CAD build for the part. Positions are in the model's coordinates, mm. A direction names the side the tool comes from. Coordinates: 2 decimals unless noted, no trailing zeros. Order: outer loops, then holes, each group sorted by start corner. A loop starts at its lowest first (then second) coordinate and runs counter-clockwise, first axis right, second up. Notation, with made-up numbers: M -31.75,88 L 1.25,88 A11 cw 1.25,98 Z; hole C 80,22 d8. An arc over 180 degrees is marked long. Write item = value, one per line. Start each with the question number.
```python
from build123d import *

# Parameters (mm, degrees)
SKETCH1_W           = 170
SKETCH1_H           = 120
BOSS_EXTRUDE1_DEPTH = 10
SKETCH2_W           = 60
SKETCH2_H           = 40
BOSS_EXTRUDE2_DEPTH = 2
SKETCH3_W           = 60
SKETCH3_H           = 8
BOSS_EXTRUDE3_DEPTH = 25
SKETCH4_R           = 1.6
CUT_EXTRUDE1_DEPTH  = 10
CUT_EXTRUDE2_DEPTH  = 36
CHAMFER1_SIZE       = 12
FILLET4_R           = 4
CHAMFER2_SIZE       = 3
CUT_EXTRUDE4_DEPTH  = 5
CUT_EXTRUDE5_DEPTH  = 19
FILLET5_R           = 10
CUT_EXTRUDE6_DEPTH  = 91
FILLET6_R           = 10


with BuildPart() as part:
    # Sketch1 → Boss-Extrude1 (new body)
    with BuildSketch(Plane(origin=(0, 0, 0), x_dir=(1, 0, 0), z_dir=(0, 1, 0))):
        with Locations((85, 60)):
            Rectangle(SKETCH1_W, SKETCH1_H)
    extrude(amount=BOSS_EXTRUDE1_DEPTH)

    # Sketch2 → Boss-Extrude2 (add)
    with BuildSketch(Plane(origin=(0, 10, 0), x_dir=(1, 0, 0), z_dir=(0, 1, 0))):
        with Locations((140, 100)):
            Rectangle(SKETCH2_W, SKETCH2_H)
    extrude(amount=BOSS_EXTRUDE2_DEPTH)

    # Sketch3 → Boss-Extrude3 (add)
    with BuildSketch(Plane(origin=(0, 12, 0), x_dir=(1, 0, 0), z_dir=(0, 1, 0))):
        with Locations((140, 84)):
            Rectangle(SKETCH3_W, SKETCH3_H)
    extrude(amount=BOSS_EXTRUDE3_DEPTH)

    # Sketch4 → Cut-Extrude1 (cut)
    with BuildSketch(Plane(origin=(0, 0, -88), x_dir=(-1, 0, 0), z_dir=(0, 0, -1))):
        with Locations((-132.854949503, 27)):
            Circle(SKETCH4_R)
        with Locations((-122.854949503, 27)):
            Circle(SKETCH4_R)
    extrude(amount=-CUT_EXTRUDE1_DEPTH, mode=Mode.SUBTRACT)

    # Sketch5 → Cut-Extrude2 (cut)
    with BuildSketch(Plane(origin=(0, 10, 0), x_dir=(1, 0, 0), z_dir=(0, 1, 0))):
        with BuildLine():
            ThreePointArc((44.934842869, 94), (84.443103198, 34.871709919), (154.189676865, 48.745166004))
            ThreePointArc((154.189676865, 48.745166004), (154.189676865, 51.573593129), (151.361249741, 51.573593129))
            ThreePointArc((151.361249741, 51.573593129), (85.973836928, 38.567228049), (48.934842869, 94))
            ThreePointArc((48.934842869, 94), (46.934842869, 96), (44.934842869, 94))
        make_face()
        with BuildLine():
            ThreePointArc((58.934842869, 94), (89.800671251, 47.806023374), (144.290181929, 58.644660941))
            ThreePointArc((144.290181929, 58.644660941), (147.118609054, 58.644660941), (147.118609054, 55.816233816))
            ThreePointArc((147.118609054, 55.816233816), (88.269937522, 44.110505244), (54.934842869, 94))
            ThreePointArc((54.934842869, 94), (56.934842869, 96), (58.934842869, 94))
        make_face()
    extrude(amount=-CUT_EXTRUDE2_DEPTH, mode=Mode.SUBTRACT)

    # Chamfer1
    chamfer1_edges = [part.edges().sort_by_distance(p)[0] for p in [
        (140, 10, -80),
    ]]
    chamfer(chamfer1_edges, length=CHAMFER1_SIZE)

    # Fillet4
    fillet4_edges = [part.edges().sort_by_distance(p)[0] for p in [
        (170, 37, -84),
        (110, 37, -84),
    ]]
    fillet(fillet4_edges, radius=FILLET4_R)

    # Chamfer2
    chamfer2_edges = [part.edges().sort_by_distance(p)[0] for p in [
        (140, 12, -88),
    ]]
    chamfer(chamfer2_edges, length=CHAMFER2_SIZE)

    # Sketch7 → Cut-Extrude4 (cut)
    with BuildSketch(Plane.XZ):
        with BuildLine():
            ThreePointArc((140.754648023, -62.180194847), (91.714088413, -52.425421037), (63.934842869, -94))
            ThreePointArc((63.934842869, -94), (51.934842869, -106), (39.934842869, -94))
            ThreePointArc((39.934842869, -94), (82.529686036, -30.252312257), (157.725210771, -45.209632098))
            ThreePointArc((157.725210771, -45.209632098), (157.725210771, -62.180194847), (140.754648023, -62.180194847))
        make_face()
    extrude(amount=-CUT_EXTRUDE4_DEPTH, mode=Mode.SUBTRACT)

    # Sketch8 → Cut-Extrude5 (cut)
    with BuildSketch(Plane(origin=(0, 10, 0), x_dir=(1, 0, 0), z_dir=(0, 1, 0))):
        Polygon((0, 0), (30, 0), (170, 0), (170, 20), (30, 20), (30, 120), (0, 120), align=None)
    extrude(amount=-CUT_EXTRUDE5_DEPTH, mode=Mode.SUBTRACT)

    # Fillet5
    fillet5_edges = [part.edges().sort_by_distance(p)[0] for p in [
        (30, 5, -120),
        (170, 5, -20),
        (110, 11, -120),
        (30, 5, -20),
        (170, 6, -120),
    ]]
    fillet(fillet5_edges, radius=FILLET5_R)

    # Sketch9 → Cut-Extrude6 (cut)
    with BuildSketch(Plane(origin=(0, 37, 0), x_dir=(1, 0, 0), z_dir=(0, 1, 0))):
        Polygon((170, 88), (170, 87), (110, 87), (110, 138.435407066), (206.694052757, 135.310318366), align=None)
    extrude(amount=-CUT_EXTRUDE6_DEPTH, mode=Mode.SUBTRACT)

    # Fillet6
    fillet6_edges = [part.edges().sort_by_distance(p)[0] for p in [
        (110, 5, -87),
        (110, 5, -120),
    ]]
    fillet(fillet6_edges, radius=FILLET6_R)


solid = part.part
```
1. Probe L1, parallel to X at y = 6, z = -62; L2, parallel to Z at x = 126, y = 7; L3, parallel to Y at x = 48, z = -49.5. List the from-to ranges inside material, lowest first.
2. Flat gauge pins, fed straight in: pin 1 (11 mm diameter, centred on y = 3.5, z = -103.5, fed in from +X); pin 2 (4.5 mm diameter, centred on x = 142, y = 27, fed in from +Z); pin 3 (5.5 mm diameter, centred on y = 20, z = -75, fed in from -X). Where does each tip first touch, or does it go through?
3. Slice it at A-A (z = -84). Write the cut outline in (x, y), plus the area to 3 significant figures.
4. Mould opens along Z. For faces 4 (the flat face through (92, 5, -50)), 5 (the cylindrical face through (57, 8, -96)), 6 (the cylindrical face through (121.33, 27.48, -83.55)), 7 (the cylindrical face through (167.15, 4.93, -23.01)) say: released by +Z, released by -Z, zero draft, split by the parting line, or undercut.
5. 3-axis set-ups, long thin cutter, end or side, ignore diameter. For faces 1 (the cylindrical face through (47, 8, -96)), 2 (the cylindrical face through (157.9, 2.5, -62)), 3 (the flat face through (110, 5, -103)): which of +Z, -Z, +X, -X, +Y, -Y reach the whole face in a straight line?
6. Slice it at C-C (x = 80). Write the cut outline in (y, z).
7. Slice it at B-B (y = 27). Write the cut outline in (x, z).
8. Slice it at D-D (y = 18). Write the cut outline in (x, z), plus the area to 3 significant figures.
Calculated:
q1.L1 = 30 to 53.51, 58.18 to 65.44, 70.52 to 170
q1.L2 = -87 to -47, -42.77 to -36.48, -32.32 to -20
q1.L3 = 0 to 10
q2.pin_1 = 110
q2.pin_2 = -80
q2.pin_3 = 110
q3.outline = M 30,0 L 40.66,0 L 40.66,5 L 45.72,5 L 45.72,10 L 30,10 Z; M 49.77,5 L 55.87,5 L 55.87,10 L 49.77,10 Z; M 59.95,5 L 65.06,5 L 65.06,0 L 170,0 L 170,33 A4 ccw 166,37 L 114,37 A4 ccw 110,33 L 110,10 L 59.95,10 Z; hole C 122.85,27 d3.2; hole C 132.85,27 d3.2
q3.area = 2,830 mm²
q4.face_4 = undercut
q4.face_5 = undercut
q4.face_6 = zero draft
q4.face_7 = released by +Z
q5.face_1 = +Y, -Y
q5.face_2 = -Y
q5.face_3 = -Z, +X, +Y, -Y
q6.outline = M 0,-120 L 10,-120 L 10,-53.22 L 5,-53.22 L 5,-59.54 L 0,-59.54 Z; M 0,-31.36 L 5,-31.36 L 5,-36.91 L 10,-36.91 L 10,-20 L 0,-20 Z; M 5,-48.41 L 10,-48.41 L 10,-41.44 L 5,-41.44 Z
q7.outline = M 110,-87 L 121.25,-87 L 121.25,-80 L 110,-80 Z; M 124.45,-87 L 131.25,-87 L 131.25,-80 L 124.45,-80 Z; M 134.45,-87 L 170,-87 L 170,-80 L 134.45,-80 Z
q8.outline = M 110,-87 L 170,-87 L 170,-76 L 110,-76 Z
q8.area = 660 mm²
